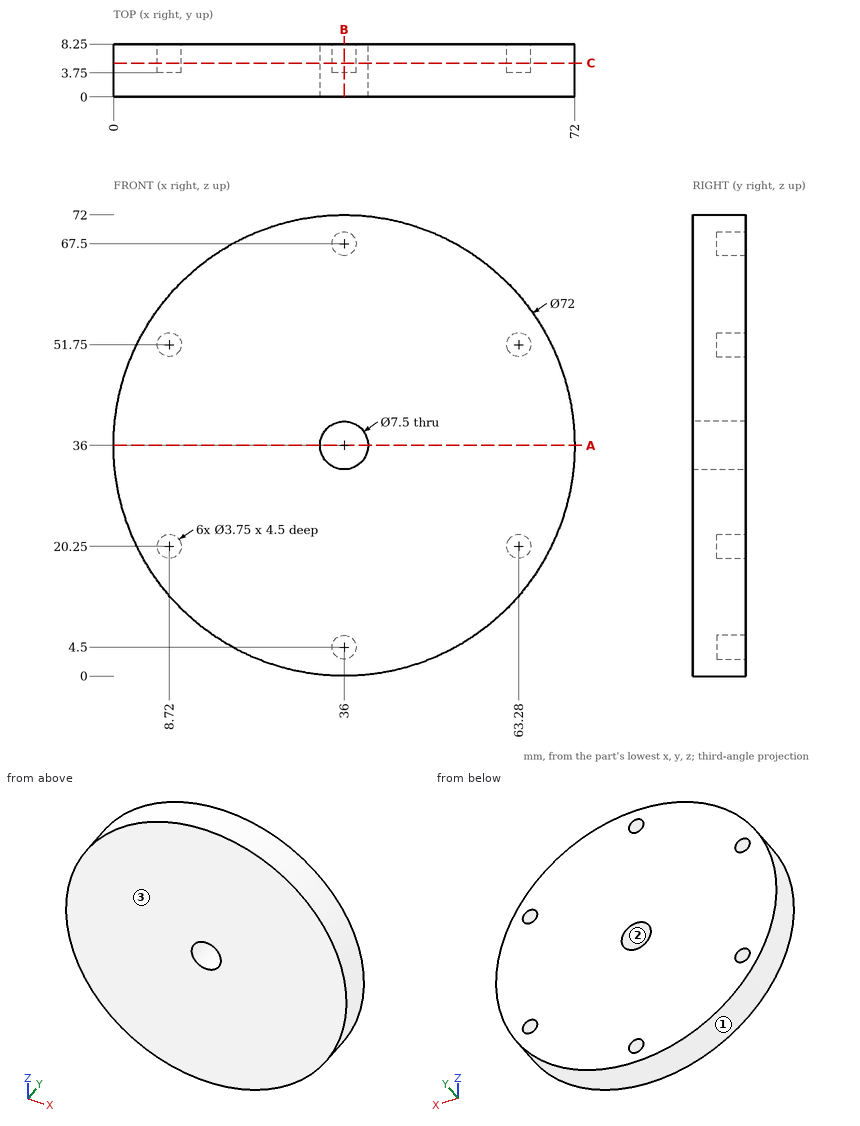
Geometry check sheet. Reference: drawing and pictorial views, mm from the part's lowest x, y, z. Give positions to 0.01 mm unless a question says otherwise; leave off trailing zeros. Order: outer loops, then holes, each group sorted by start corner. A loop starts at its lowest first (then second) coordinate and runs counter-clockwise, first axis right, second up.
1. Section check B-B, the plane x = 36. Enter the section's corners in (y, z) (3 decimals).
2. Gauge pin test, flat ends, axial feed: pin 1 Ø6 at (x, z) = (36, 36) entering from +Y; pin 2 Ø1.1 at (x, z) = (37, 67.5) entering from +Y; pin 3 Ø4 at (x, z) = (62.5, 20.5) entering from +Y; pin 4 Ø1 at (y, z) = (5.5, 29.5) entering from +X. Record the tip position at first contact, or that the pin passes through.
3. Section check A-A, the plane z = 36. Enter the section's corners in (x, y).
4. Release check for a two-part mould opening along X. For the marked faces 1, 2 and 3 record: pulls with the +X half, pulls with the -X half, needs draft (parallel to the pull), parting line crosses it, or undercut.
5. Section check C-C, the plane y = 5.25. Give the number of separate pieces and of enclosed holes in the cut face, and give its area (3 significant figures).
6. Thickness scan on L1, parallel to X at y = 6.5, z = 53; L2, parallel to X at y = 7.15, z = 51.75 (1 decimal); L3, parallel to X at y = 5.5, z = 4.5 (1 decimal). Record the ranges inside material, lowest first.
Values follow:
1. outline: (0, 0) - (8.25, 0) - (8.25, 2.625) - (3.75, 2.625) - (3.75, 6.375) - (8.25, 6.375) - (8.25, 32.25) - (0, 32.25) - close; (0, 39.75) - (8.25, 39.75) - (8.25, 65.625) - (3.75, 65.625) - (3.75, 69.375) - (8.25, 69.375) - (8.25, 72) - (0, 72) - close
2. pin 1: passes through
2. pin 2: stops at y = 3.75
2. pin 3: stops at y = 8.25
2. pin 4: stops at x = 71.5
3. outline: (0, 0) - (32.25, 0) - (32.25, 8.25) - (0, 8.25) - close; (39.75, 0) - (72, 0) - (72, 8.25) - (39.75, 8.25) - close
4. face 1: parting line crosses it
4. face 2: undercut
4. face 3: needs draft
5. separate pieces: 1
5. enclosed holes: 7
5. area: 3,960 mm2
6. L1: x = 4.27 to 7.32, 10.12 to 61.88, 64.68 to 67.73
6. L2: x = 3.6 to 6.8, 10.6 to 61.4, 65.2 to 68.4
6. L3: x = 18.6 to 34.1, 37.9 to 53.4
